Autodesk Inventor part; units mm, degrees
ref_plane "YZ Plane" through (0, 0, 0) normal (1, 0, 0) x (0, 1, 0)
ref_plane "XZ Plane" through (0, 0, 0) normal (0, 1, 0) x (-1, 0, 0)
ref_plane "XY Plane" through (0, 0, 0) normal (0, 0, 1) x (1, 0, 0)
sketch "スケッチ1" plane through (0, 0, 0) normal (0, 0, 1) x (1, 0, 0)
  line L0 (0, 0) -> (11.7, 0)
  line L1 (11.7, 0) -> (11.7, 22.7)
  line L2 (11.7, 22.7) -> (0, 22.7)
  line L3 (0, 22.7) -> (0, 0)
  dimension "d0" = 11.7
  dimension "d1" = 22.7
extrude "押し出し1" add sketch "スケッチ1" along normal blind 20.7
sketch "スケッチ2" plane through (0, 0, 20.7) normal (0, 0, 1) x (1, 0, 0)
  line L0 (11.7, 22.7) -> (0, 22.7)
  arc A0 (2.9453, 11.45) -> (8.7547, 11.45) centre (5.85, 10.7) ccw
  line L1 (0, 22.7) -> (0, 0)
  line L2 (11.7, 0) -> (11.7, 22.7)
  arc A1 (0, 15.3668) -> (2.9453, 11.45) centre (5.85, 16.7) ccw
  arc A2 (8.7547, 11.45) -> (11.7, 15.3668) centre (5.85, 16.7) ccw
  arc A3 (11.7, 18.0332) -> (0, 18.0332) centre (5.85, 16.7) ccw
  dimension "d5" = 6
  dimension "d6" = 6
extrude "押し出し2" add sketch "スケッチ2" along normal blind 2.5 contours A3 L2 A2 A0 A1 L1
sketch "スケッチ3" plane through (0, 0, 23.2) normal (0, 0, 1) x (1, 0, 0)
  arc A0 (11.7, 18.0332) -> (0, 18.0332) centre (5.85, 16.7) ccw
  circle A1 centre (5.85, 16.7) radius 2
  point P0 (0, 0)
  dimension "d9" = 4
extrude "押し出し3" add sketch "スケッチ3" along normal blind 2.5
sketch "スケッチ4" plane through (0, 0, 0) normal (0, -1, 0) x (1, 0, 0)
  line L0 (11.7, 0) -> (11.7, 20.7)
  line L1 (0, 17.7) -> (11.7, 17.7)
  line L2 (11.7, 17.7) -> (11.7, 16.7)
  line L3 (11.7, 16.7) -> (0, 16.7)
  line L4 (0, 16.7) -> (0, 17.7)
  point P0 (0, 0)
  dimension "d12" = 1
extrude "押し出し4" add sketch "スケッチ4" along normal blind 4.5
sketch "スケッチ5" plane through (0, 22.7, 0) normal (0, 1, 0) x (1, 0, 0)
  line L0 (11.7, -17.7) -> (11.7, -20.7)
  line L1 (11.7, -17.7) -> (0, -17.7)
  line L2 (0, -17.7) -> (0, -16.7)
  line L3 (0, -16.7) -> (11.7, -16.7)
  line L4 (11.7, -16.7) -> (11.7, -17.7)
  point P0 (0, 0)
  dimension "d15" = 1
extrude "押し出し5" add sketch "スケッチ5" along normal blind 4.5
sketch "スケッチ6" plane through (0, 0, 17.7) normal (0, 0, 1) x (1, 0, 0)
  line L0 (0, -4.5) -> (11.7, -4.5)
  line L1 (2, -4.5) -> (1, 0)
  line L2 (0, 0) -> (11.7, 0)
  line L3 (10.7, 0) -> (9.7, -4.5)
  line L4 (0, 27.2) -> (11.7, 27.2)
  line L5 (5.85, 22.7) -> (0, 22.7)
  line L6 (1.5, 22.7) -> (2, 27.2)
  line L7 (11.7, 22.7) -> (0, 22.7)
  line L8 (10.7, 22.7) -> (9.7, 27.2)
  circle A0 centre (5.85, 25.7) radius 1
  circle A1 centre (5.85, -2.5) radius 1
  line L9 (11.7, -4.5) -> (11.7, 0)
  line L10 (0, 0) -> (0, -4.5)
  line L11 (0, 22.7) -> (0, 27.2)
  line L12 (11.7, 27.2) -> (11.7, 22.7)
  line L13 (0, -4.5) -> (0, 0)
  line L14 (11.7, 0) -> (11.7, -4.5)
  line L15 (0, 22.7) -> (0, 27.2)
  line L16 (11.7, 27.2) -> (11.7, 22.7)
  line L17 (11.7, -4.5) -> (9.7, -4.5)
  line L18 (2, -4.5) -> (0, -4.5)
  line L19 (0, 0) -> (1, 0)
  line L20 (10.7, 0) -> (11.7, 0)
  line L21 (11.7, 22.7) -> (10.7, 22.7)
  line L22 (1.5, 22.7) -> (0, 22.7)
  line L23 (0, 27.2) -> (2, 27.2)
  line L24 (9.7, 27.2) -> (11.7, 27.2)
  dimension "d18" = 2
  dimension "d19" = 2
extrude "押し出し6" cut sketch "スケッチ6" against normal blind 4.5 contours L10 L2 L1 L0 | L3 L2 L9 L0 | L4 L6 L5 L11 | L4 L12 L7 L8 | A0 | A1
sketch "スケッチ7" plane through (0, 22.7, 0) normal (0, 1, 0) x (1, 0, 0)
  line L0 (3.1, -2.5) -> (8.6, -2.5)
  line L1 (8.6, -2.5) -> (8.6, -5.5)
  line L2 (8.6, -5.5) -> (3.1, -5.5)
  line L3 (3.1, -5.5) -> (3.1, -2.5)
  line L4 (0, 0) -> (0, -20.7)
  dimension "d22" = 5.5
  dimension "d23" = 3
extrude "押し出し7" add sketch "スケッチ7" along normal blind 3
properties part number "RB-001-Servo" material "ABS プラスチック"
Here's how the part is built. I have some questions about the finished solid (model axes, mm). A direction names the side the tool comes from. Give positions to 0.01 mm unless a question says otherwise; leave off trailing zeros. Write each loop counter-clockwise with the first axis right and the second up, starting at its lowest first coordinate (ties: lowest second). Pieces come first, ordered by that corner, then holes. Notation, with made-up numbers: (73, -14.75) -> (87, -14.75) arc R24 ccw to (87, 21.25) -> close; hole circle Ø6 at (72.25, 86). An arc over 180 degrees is marked (long way). Use one line per item in the form item = value. Start each with the question number.
1. Imagine slicing it at C-C on x = 5.5. State how many separate pieces and enclosed holes the cut face has, plus the area to 3 significant figures.
2. Imagine slicing it at D-D on y = -2.5. List the corners of the cut face in (x, z) for me, plus the area to 3 significant figures.
3. If I drill on L1, parallel to Y at x = 5.85, z = 17.45; L2, parallel to Y at x = 7.25, z = 13.25; L3, parallel to Z at x = 7.25, y = 26, over which ranges is the centre line in solid material (lowest first)?
4. Thinking about a two-plate mould opening in Z: for faces 1 (the face through (0, 12, 11)), 2 (the face through (6, 22.7, 10)), 3 (the face through (6, 14, 23.2)), which applies, +Z half, -Z half, draft (parallel to the pull), parting line (faces both ways), or undercut?
5. Imagine slicing it at B-B on z = 3.25. List the corners of the cut face in (x, y) for me, plus the area to 3 significant figures.
6. On a 3-axis mill with a long thin cutter (end or side, diameter ignored), from which of +Z, -Z, +X, -X, +Y, -Y can I reach the whole of each face in a straight line? I mean faces 4 (the face through (10, 22, 20.7)), 5 (the face through (6, 24, 16.7)), 6 (the face through (8.6, 24, 4)). Say none if no direction works.
7. Will these pins go through, and if not, where does the flat tip stop? pin 1 Ø2.5 at (x, y) = (6, 24.5) entering from +Z; pin 2 Ø1.6 at (x, y) = (5.85, -2.5) entering from +Z; pin 3 Ø1 at (x, y) = (10, 21.5) entering from +Z; pin 4 Ø1.5 at (x, z) = (7, 4) entering from +Y.
8. Imagine slicing it at A-A on y = 10.7. List the corners of the cut face in (x, z) for me.
Entries:
q1.separate_pieces = 3
q1.enclosed_holes = 0
q1.area = 531 mm²
q2.outline = (1.56, 16.7) -> (4.85, 16.7) -> (4.85, 17.7) -> (1.56, 17.7) -> close; (6.85, 16.7) -> (10.14, 16.7) -> (10.14, 17.7) -> (6.85, 17.7) -> close
q2.area = 6.59 mm²
q3.L1 = -4.5 to -3.5, -1.5 to 24.7, 26.7 to 27.2
q3.L2 = 0 to 22.7
q3.L3 = 16.7 to 17.7
q4.face_1 = draft
q4.face_2 = undercut
q4.face_3 = +Z half
q5.outline = (0, 0) -> (11.7, 0) -> (11.7, 22.7) -> (8.6, 22.7) -> (8.6, 25.7) -> (3.1, 25.7) -> (3.1, 22.7) -> (0, 22.7) -> close
q5.area = 282 mm²
q6.face_4 = +Z, +X, +Y
q6.face_5 = +X, -X, +Y
q6.face_6 = -Z, +X, +Y
q7.pin_1 = 17.7
q7.pin_2 = through
q7.pin_3 = 23.2
q7.pin_4 = 25.7
q8.outline = (0, 0) -> (11.7, 0) -> (11.7, 20.7) -> (8.85, 20.7) -> (8.85, 23.2) -> (2.85, 23.2) -> (2.85, 20.7) -> (0, 20.7) -> close
